Build history of the part. All positions in model axes, mm. Face numbers are marked on the shaded views. A direction names the side the tool comes from. Coordinates: 2 decimals unless noted, no trailing zeros.
(1) Slice it at A-A (x = 22.5). Give the number of separate pieces and of enclosed holes in the cut face, and give its area (3 significant figures).
(2) Tool access for the marked faces 1, 2, 3, 4 and 5: list every direction of +Z, -Z, +X, -X, +Y, -Y with a clear straight run to the whole face (end or side of a thin tool).
(3) Flat gauge pins, fed straight in: P1, Ø6, axis at x = 22.5, y = 16.75, coming from the +Z side; P2, Ø5, axis at y = 0, z = 8, coming from the +X side; P3, Ø5, axis at x = 0.5, y = -13.5, coming from the +Z side. Where does each tip first touch, or does it go through?
(4) Wall check: L1, parallel to Y at x = -23.5, z = -8.5; L2, parallel to X at y = -18.5, z = -4.5; L3, parallel to Z at x = -3.5, y = -14. Give the ranges that are in metal, low to high.
(5) Two-plate mould, pull along Y, no slides. Class the marked faces 6, 7 and 8: pulls with the +Y half, pulls with the -Y half, needs draft (parallel to the pull), parting line crosses it, or undercut.
from build123d import *

# Parameters (mm, degrees)
SKETCH2_R           = 5.25
BOSS_EXTRUDE1_DEPTH = 30
SKETCH4_R           = 11.5
CUT_EXTRUDE1_DEPTH  = 30
CUT_EXTRUDE2_REACH  = 42.716
SKETCH5_R           = 1.75
SKETCH6_R           = 2.65
CUT_EXTRUDE3_DEPTH  = 5.3
CUT_EXTRUDE4_REACH  = 50.771
SKETCH8_R           = 2.25
CUT_EXTRUDE6_REACH  = 68.014
SKETCH10_W          = 7.5
SKETCH10_H          = 12
CUT_EXTRUDE5_DEPTH  = 3
FILLET2_R           = 2.4
FILLET3_R           = 7.4


with BuildPart() as part:
    # Sketch2 → Boss-Extrude1 (new, symmetric)
    with BuildSketch(Plane(origin=(0, 0, 0), x_dir=(0, 0, -1), z_dir=(1, 0, 0))):
        Polygon((-15.5, 22.75), (-15.5, -22.75), (10.5, -22.75), (10.5, -7), (15.5, -7), (15.5, 7), (10.5, 7), (10.5, 22.75), align=None)
        Circle(SKETCH2_R, mode=Mode.SUBTRACT)
    extrude(amount=BOSS_EXTRUDE1_DEPTH, both=True)

    # Sketch4 → Cut-Extrude1 (cut)
    with BuildSketch(Plane.ZY.offset(30)):
        Circle(SKETCH4_R)
    extrude(amount=-CUT_EXTRUDE1_DEPTH, mode=Mode.SUBTRACT)

    # Sketch5 → Cut-Extrude2 (cut, up to next)
    with BuildSketch(Plane.ZY, mode=Mode.PRIVATE) as cut_extrude2_sk1:
        with Locations((0, 8)):
            Circle(SKETCH5_R)
    cut_extrude2_tool1 = extrude(cut_extrude2_sk1.sketch, amount=-CUT_EXTRUDE2_REACH, mode=Mode.PRIVATE) & part.part
    # Sketch5 → Cut-Extrude2 (cut, up to next)
    with BuildSketch(Plane.ZY, mode=Mode.PRIVATE) as cut_extrude2_sk2:
        with Locations((8, 0)):
            Circle(SKETCH5_R)
    cut_extrude2_tool2 = extrude(cut_extrude2_sk2.sketch, amount=-CUT_EXTRUDE2_REACH, mode=Mode.PRIVATE) & part.part
    # Sketch5 → Cut-Extrude2 (cut, up to next)
    with BuildSketch(Plane.ZY, mode=Mode.PRIVATE) as cut_extrude2_sk3:
        with Locations((0, -8)):
            Circle(SKETCH5_R)
    cut_extrude2_tool3 = extrude(cut_extrude2_sk3.sketch, amount=-CUT_EXTRUDE2_REACH, mode=Mode.PRIVATE) & part.part
    # Sketch5 → Cut-Extrude2 (cut, up to next)
    with BuildSketch(Plane.ZY, mode=Mode.PRIVATE) as cut_extrude2_sk4:
        with Locations((-8, 0)):
            Circle(SKETCH5_R)
    cut_extrude2_tool4 = extrude(cut_extrude2_sk4.sketch, amount=-CUT_EXTRUDE2_REACH, mode=Mode.PRIVATE) & part.part
    add(cut_extrude2_tool1.solids().sort_by_distance((0, 8, 0))[0], mode=Mode.SUBTRACT)
    add(cut_extrude2_tool2.solids().sort_by_distance((0, 0, 8))[0], mode=Mode.SUBTRACT)
    add(cut_extrude2_tool3.solids().sort_by_distance((0, -8, 0))[0], mode=Mode.SUBTRACT)
    add(cut_extrude2_tool4.solids().sort_by_distance((0, 0, -8))[0], mode=Mode.SUBTRACT)

    # Sketch6 → Cut-Extrude3 (cut)
    with BuildSketch(Plane(origin=(30, 0, 0), x_dir=(0, 0, -1), z_dir=(1, 0, 0))):
        with Locations((0, 8)):
            Circle(SKETCH6_R)
        with Locations((8, 0)):
            Circle(SKETCH6_R)
        with Locations((0, -8)):
            Circle(SKETCH6_R)
        with Locations((-8, 0)):
            Circle(SKETCH6_R)
    extrude(amount=-CUT_EXTRUDE3_DEPTH, mode=Mode.SUBTRACT)

    # Sketch8 → Cut-Extrude4 (cut, up to next)
    with BuildSketch(Plane.XY.offset(15.5), mode=Mode.PRIVATE) as cut_extrude4_sk1:
        with Locations((-22.5, 16.75)):
            Circle(SKETCH8_R)
    cut_extrude4_tool1 = extrude(cut_extrude4_sk1.sketch, amount=-CUT_EXTRUDE4_REACH, mode=Mode.PRIVATE) & part.part
    # Sketch8 → Cut-Extrude4 (cut, up to next)
    with BuildSketch(Plane.XY.offset(15.5), mode=Mode.PRIVATE) as cut_extrude4_sk2:
        with Locations((-7.5, 16.75)):
            Circle(SKETCH8_R)
    cut_extrude4_tool2 = extrude(cut_extrude4_sk2.sketch, amount=-CUT_EXTRUDE4_REACH, mode=Mode.PRIVATE) & part.part
    # Sketch8 → Cut-Extrude4 (cut, up to next)
    with BuildSketch(Plane.XY.offset(15.5), mode=Mode.PRIVATE) as cut_extrude4_sk3:
        with Locations((7.5, 16.75)):
            Circle(SKETCH8_R)
    cut_extrude4_tool3 = extrude(cut_extrude4_sk3.sketch, amount=-CUT_EXTRUDE4_REACH, mode=Mode.PRIVATE) & part.part
    # Sketch8 → Cut-Extrude4 (cut, up to next)
    with BuildSketch(Plane.XY.offset(15.5), mode=Mode.PRIVATE) as cut_extrude4_sk4:
        with Locations((22.5, 16.75)):
            Circle(SKETCH8_R)
    cut_extrude4_tool4 = extrude(cut_extrude4_sk4.sketch, amount=-CUT_EXTRUDE4_REACH, mode=Mode.PRIVATE) & part.part
    # Sketch8 → Cut-Extrude4 (cut, up to next)
    with BuildSketch(Plane.XY.offset(15.5), mode=Mode.PRIVATE) as cut_extrude4_sk5:
        with Locations(Location((22.5, -16.75, 0), (0, 0, 270))):
            Circle(SKETCH8_R)
    cut_extrude4_tool5 = extrude(cut_extrude4_sk5.sketch, amount=-CUT_EXTRUDE4_REACH, mode=Mode.PRIVATE) & part.part
    # Sketch8 → Cut-Extrude4 (cut, up to next)
    with BuildSketch(Plane.XY.offset(15.5), mode=Mode.PRIVATE) as cut_extrude4_sk6:
        with Locations(Location((7.5, -16.75, 0), (0, 0, 270))):
            Circle(SKETCH8_R)
    cut_extrude4_tool6 = extrude(cut_extrude4_sk6.sketch, amount=-CUT_EXTRUDE4_REACH, mode=Mode.PRIVATE) & part.part
    # Sketch8 → Cut-Extrude4 (cut, up to next)
    with BuildSketch(Plane.XY.offset(15.5), mode=Mode.PRIVATE) as cut_extrude4_sk7:
        with Locations(Location((-7.5, -16.75, 0), (0, 0, 270))):
            Circle(SKETCH8_R)
    cut_extrude4_tool7 = extrude(cut_extrude4_sk7.sketch, amount=-CUT_EXTRUDE4_REACH, mode=Mode.PRIVATE) & part.part
    # Sketch8 → Cut-Extrude4 (cut, up to next)
    with BuildSketch(Plane.XY.offset(15.5), mode=Mode.PRIVATE) as cut_extrude4_sk8:
        with Locations(Location((-22.5, -16.75, 0), (0, 0, 270))):
            Circle(SKETCH8_R)
    cut_extrude4_tool8 = extrude(cut_extrude4_sk8.sketch, amount=-CUT_EXTRUDE4_REACH, mode=Mode.PRIVATE) & part.part
    add(cut_extrude4_tool1.solids().sort_by_distance((-22.5, 16.75, 15.5))[0], mode=Mode.SUBTRACT)
    add(cut_extrude4_tool2.solids().sort_by_distance((-7.5, 16.75, 15.5))[0], mode=Mode.SUBTRACT)
    add(cut_extrude4_tool3.solids().sort_by_distance((7.5, 16.75, 15.5))[0], mode=Mode.SUBTRACT)
    add(cut_extrude4_tool4.solids().sort_by_distance((22.5, 16.75, 15.5))[0], mode=Mode.SUBTRACT)
    add(cut_extrude4_tool5.solids().sort_by_distance((22.5, -16.75, 15.5))[0], mode=Mode.SUBTRACT)
    add(cut_extrude4_tool6.solids().sort_by_distance((7.5, -16.75, 15.5))[0], mode=Mode.SUBTRACT)
    add(cut_extrude4_tool7.solids().sort_by_distance((-7.5, -16.75, 15.5))[0], mode=Mode.SUBTRACT)
    add(cut_extrude4_tool8.solids().sort_by_distance((-22.5, -16.75, 15.5))[0], mode=Mode.SUBTRACT)

    # Sketch10 → Cut-Extrude6 (cut, up to next)
    with BuildSketch(Plane(origin=(30, 0, 0), x_dir=(0, 0, -1), z_dir=(1, 0, 0)), mode=Mode.PRIVATE) as cut_extrude6_sk1:
        with Locations((-11.75, 16.75)):
            Rectangle(SKETCH10_W, SKETCH10_H)
    cut_extrude6_tool1 = extrude(cut_extrude6_sk1.sketch, amount=-CUT_EXTRUDE6_REACH, mode=Mode.PRIVATE) & part.part
    # Sketch10 → Cut-Extrude6 (cut, up to next)
    with BuildSketch(Plane(origin=(30, 0, 0), x_dir=(0, 0, -1), z_dir=(1, 0, 0)), mode=Mode.PRIVATE) as cut_extrude6_sk2:
        with Locations((-11.75, -16.75)):
            Rectangle(SKETCH10_W, SKETCH10_H)
    cut_extrude6_tool2 = extrude(cut_extrude6_sk2.sketch, amount=-CUT_EXTRUDE6_REACH, mode=Mode.PRIVATE) & part.part
    add(cut_extrude6_tool1.solids().sort_by_distance((30, 16.75, 11.75))[0], mode=Mode.SUBTRACT)
    add(cut_extrude6_tool2.solids().sort_by_distance((30, -16.75, 11.75))[0], mode=Mode.SUBTRACT)

    # Sketch9 → Cut-Extrude5 (cut)
    with BuildSketch(Plane.XY.offset(8)):
        Polygon((-3.343078062, 16.75), (-5.421539031, 20.35), (-9.578460969, 20.35), (-11.656921938, 16.75), (-9.578460969, 13.15), (-5.421539031, 13.15), align=None)
        Polygon((-18.343078062, 16.75), (-20.421539031, 20.35), (-24.578460969, 20.35), (-26.656921938, 16.75), (-24.578460969, 13.15), (-20.421539031, 13.15), align=None)
        Polygon((11.656921938, 16.75), (9.578460969, 20.35), (5.421539031, 20.35), (3.343078062, 16.75), (5.421539031, 13.15), (9.578460969, 13.15), align=None)
        Polygon((26.656921938, 16.75), (24.578460969, 20.35), (20.421539031, 20.35), (18.343078062, 16.75), (20.421539031, 13.15), (24.578460969, 13.15), align=None)
        Polygon((24.578460969, -13.15), (26.656921938, -16.75), (24.578460969, -20.35), (20.421539031, -20.35), (18.343078062, -16.75), (20.421539031, -13.15), align=None)
        Polygon((9.578460969, -13.15), (11.656921938, -16.75), (9.578460969, -20.35), (5.421539031, -20.35), (3.343078062, -16.75), (5.421539031, -13.15), align=None)
        Polygon((-5.421539031, -13.15), (-3.343078062, -16.75), (-5.421539031, -20.35), (-9.578460969, -20.35), (-11.656921938, -16.75), (-9.578460969, -13.15), align=None)
        Polygon((-20.421539031, -13.15), (-18.343078062, -16.75), (-20.421539031, -20.35), (-24.578460969, -20.35), (-26.656921938, -16.75), (-24.578460969, -13.15), align=None)
    extrude(amount=-CUT_EXTRUDE5_DEPTH, mode=Mode.SUBTRACT)

    # Fillet2
    fillet2_edges = [part.edges().sort_by_distance(p)[0] for p in [
        (0, 10.75, 8),
        (0, -10.75, 8),
    ]]
    fillet(fillet2_edges, radius=FILLET2_R - 0.0001)  # a hair under: the kernel refuses the full size

    # Fillet3
    fillet3_edges = [part.edges().sort_by_distance(p)[0] for p in [
        (0, -10.75, 15.5),
        (0, 10.75, 15.5),
    ]]
    fillet(fillet3_edges, radius=FILLET3_R)


solid = part.part
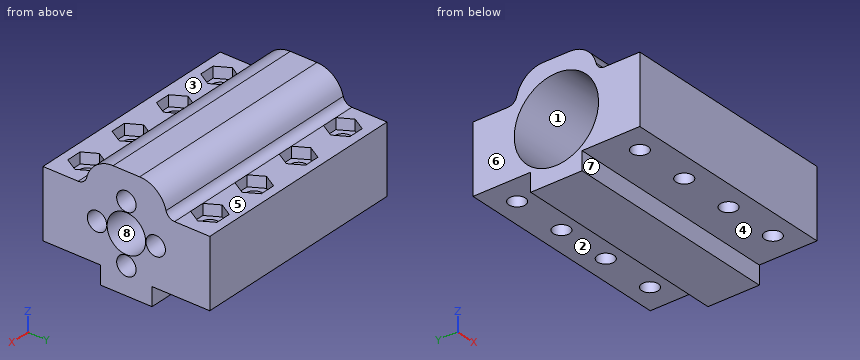
Response values:
1. separate pieces: 3
1. enclosed holes: 5
1. area: 748 mm2
2. face 1: -X
2. face 2: -Z, +X, -X, +Y
2. face 3: +Z, +X, -X, -Y
2. face 4: -Z, +X, -X, -Y
2. face 5: +Z, +X, -X, +Y
3. P1: stops at z = 5
3. P2: stops at x = 24.7
3. P3: stops at z = 9.33
4. L1: y = -22.75 to -18.77, -14.73 to -7.75, 7.75 to 14.73, 18.77 to 22.75
4. L2: x = -30 to -23.91, -21.09 to -8.91, -6.09 to 6.09, 8.91 to 21.09, 23.91 to 30
4. L3: z = -10.5 to 8
5. face 6: needs draft
5. face 7: pulls with the -Y half
5. face 8: undercut
